The model under review builds one solid part; all positions refer to its coordinate system, in mm. Face numbers are marked on the shaded views. A direction names the side the tool comes from. Round coordinates to 2 decimals unless told otherwise and drop trailing zeros. Order: outer loops, then holes, each group sorted by start corner. A loop starts at its lowest first (then second) coordinate and runs counter-clockwise, first axis right, second up. Notation, with made-up numbers: (41, 53) -> (50, 53) arc R21 ccw to (50, 60) -> close; hole circle Ø4 at (23.25, -15.5). An arc over 180 degrees is marked (long way). Return JSON: item names as keys, results as strings. Group by question number.
Autodesk Inventor part; units mm, degrees
ref_plane "YZ Plane" through (0, 0, 0) normal (1, 0, 0) x (0, 1, 0)
ref_plane "XZ Plane" through (0, 0, 0) normal (0, 1, 0) x (-1, 0, 0)
ref_plane "XY Plane" through (0, 0, 0) normal (0, 0, 1) x (1, 0, 0)
sketch "Skizze1" plane through (0, 0, 0) normal (0, 1, 0) x (-1, 0, 0)
  line L0 (0, -50) -> (-50, -50)
  line L1 (-50, -50) -> (-50, 50)
  line L2 (-50, 50) -> (0, 50)
  line L3 (0, -50) -> (50, -50)
  line L4 (50, -50) -> (50, 50)
  line L5 (50, 50) -> (0, 50)
  line L6 (-122.5, 0) -> (122.5, 0) construction
  line L7 (0, -77.2) -> (0, 113.2) construction
  dimension "d1" = 100
  dimension "d3" = 100
extrude "Grundkoerper" add sketch "Skizze1" along normal mid plane 65
sketch "Skizze2" plane through (0, -32.5, 0) normal (0, -1, 0) x (1, 0, 0)
  line L0 (-50, -50) -> (50, -50)
  line L1 (50, 50) -> (-50, 50)
  point P0 (0, 0)
  point P1 (0, 0)
  point P2 (-87.5, 0)
  point P3 (87.5, 0)
  dimension "d8" = 0
sketch "Skizze3" plane through (0, 0, 0) normal (1, 0, 0) x (0, 1, 0)
  line L0 (49, 0) -> (-49, 0) construction
  line L1 (-32.5, 50) -> (-32.5, -50) construction
  line L2 (32.5, -50) -> (32.5, 50) construction
  line L3 (32.5, 36) -> (-12.5, 36)
  line L4 (-12.5, 36) -> (-12.5, 32.25)
  line L5 (-17.5, 18) -> (-32.5, 18)
  line L6 (-32.5, -50) -> (-32.5, 50)
  line L7 (-32.5, 18) -> (-32.5, 0)
  line L8 (-32.5, 0) -> (32.5, 0)
  line L9 (32.5, 0) -> (32.5, 36)
  line L10 (-12.5, 32.25) -> (-17.5, 32.25)
  line L11 (-17.5, 32.25) -> (-17.5, 18)
  point P0 (0, 0)
  dimension "d9" = 45
  dimension "d10" = 72
  dimension "d11" = 36
  dimension "d33" = 5
  dimension "d34" = 64.5
revolve "Lagersitz" cut sketch "Skizze3" angle 360 about axis through (0, -32.5, 0) along (0, -1, 0)
sketch "Skizze_Lagersitz" plane through (0, 0, 0) normal (1, 0, 0) x (0, 1, 0)
  line L0 (-12.5, 36) -> (32.5, 36)
  line L1 (-12.5, -36) -> (-12.5, 36)
  line L2 (-17.5, 32.25) -> (-12.5, 32.25)
  line L3 (-17.5, -32.25) -> (-17.5, 32.25)
  line L4 (-32.5, 18) -> (-17.5, 18)
  line L5 (-32.5, -18) -> (-17.5, -18)
  line L6 (-17.5, -32.25) -> (-12.5, -32.25)
  line L7 (-12.5, -36) -> (32.5, -36)
  line L8 (32.5, 36) -> (32.5, -36)
  line L9 (32.5, 50) -> (32.5, -50)
  line L10 (30, -50) -> (30, 0)
  line L11 (-32.5, -18) -> (-32.5, 18)
  line L12 (-32.5, 50) -> (-32.5, -50)
  line L13 (-32.5, -50) -> (-32.5, 50)
  line L14 (-12.5, -36) -> (-12.5, 36)
  point P0 (0, 0)
  point P1 (30, 86)
  point P2 (30, 14)
  point P3 (-30, 32)
  point P4 (-30, 68)
sketch "Skizze10" plane through (0, 0, 0) normal (1, 0, 0) x (0, 1, 0)
  line L0 (49, 0) -> (-49, 0)
  line L1 (-32.5, 18) -> (-17.5, 18) construction
  line L2 (-32.5, -50) -> (-32.5, 50) construction
  line L3 (-17.5, -32.25) -> (-17.5, 32.25) construction
  line L4 (-32.5, 50) -> (-32.5, -50)
  line L5 (-29.5, 27.5) -> (-21.7, 27.5)
  line L6 (-21.2, 27) -> (-21.2, 22.5)
  line L7 (-21.2, 22.5) -> (-17.5, 22.5)
  line L8 (-17.5, 22.5) -> (-17.5, 18)
  line L9 (-32.5, 40) -> (-32.5, 0)
  line L10 (-32.5, 0) -> (-17.5, 0)
  line L11 (-17.5, 0) -> (-17.5, 22.5)
  arc A0 (-21.2, 27) -> (-21.7, 27.5) centre (-21.7, 27) ccw
  line L12 (-29.5, 27.5) -> (-29.5, 40)
  line L13 (-29.5, 40) -> (-32.5, 40)
  point P0 (0, 0)
  dimension "d117" = 55
  dimension "d118" = 0.5
  dimension "d119" = 45
  dimension "d124" = 8.3
  dimension "d125" = 3
  dimension "d126" = 80
revolve "RWDR" cut sketch "Skizze10" angle 360 about axis through (0, -32.5, 0) along (0, -1, 0)
sketch "Skizze_RWDR" plane through (0, 0, 0) normal (1, 0, 0) x (0, 1, 0)
  line L0 (-32.5, -40) -> (-32.5, 40)
  line L1 (-32.5, 40) -> (-29.5, 40)
  line L2 (-29.5, -40) -> (-29.5, 40)
  line L3 (-32.5, -40) -> (-29.5, -40)
  line L4 (-29.5, 27.5) -> (-21.7, 27.5)
  line L5 (-21.2, -27) -> (-21.2, 27)
  line L6 (-29.5, -27.5) -> (-21.7, -27.5)
  arc A0 (-21.7, -27.5) -> (-21.2, -27) centre (-21.7, -27) ccw
  arc A1 (-21.2, 27) -> (-21.7, 27.5) centre (-21.7, 27) ccw
  line L7 (-21.2, 22.5) -> (-17.5, 22.5)
  line L8 (-21.2, -22.5) -> (-17.5, -22.5)
  line L9 (-17.5, 22.5) -> (-17.5, -22.5)
  point P0 (0, 0)
sketch "Skizze5" plane through (0, 32.5, 0) normal (0, 1, 0) x (1, 0, 0)
  circle A0 centre (0, 0) radius 36 construction
  circle A1 centre (0, 0) radius 43 construction
  line L0 (-50, -50) -> (50, -50) construction
  line L1 (50, 50) -> (-50, 50)
  line L2 (-50, 50) -> (50, 50) construction
  line L3 (0, 77.2) -> (0, -113.2) construction
  line L4 (0, 0) -> (21.5, -37.2391) construction
  point P0 (43, 0)
  point P1 (21.5, 37.2391)
  point P2 (-21.5, 37.2391)
  point P3 (-43, 0)
  point P4 (-21.5, -37.2391)
  dimension "d40" = 86
  dimension "d38" = 100
  dimension "d39" = 72
  dimension "d110" = 30
  dimension "d114" = 360
hole "M6_Boh_Lagerpresse" at (21.5, 32.5, 37.2391) at (43, 32.5, 0) at (21.5, 32.5, -37.2391) at (-21.5, 32.5, -37.2391) at (-43, 32.5, 0) at (-21.5, 32.5, 37.2391) direction (0, -1, 0) diameter 4.917 depth 17.1 tip angle 118 countersink diameter 6 countersink angle 90
sketch "Skizze11" plane through (0, -29.5, 0) normal (0, -1, 0) x (1, 0, 0)
  circle A0 centre (0, 0) radius 40 construction
  circle A1 centre (0, 0) radius 27.5 construction
  circle A2 centre (0, 0) radius 33.75 construction
  line L0 (0, 113.2) -> (0, -77.2) construction
  line L1 (-122.5, 0) -> (122.5, 0)
  point P0 (0, 33.75)
  point P1 (-33.75, 0)
  point P2 (0, -33.75)
  point P3 (33.75, 0)
  dimension "d129" = 67.5
  dimension "d127" = 55
  dimension "d128" = 80
  dimension "d132" = 360
hole "M3_RWDR_Fixierung" at (0, -29.5, 33.75) at (-33.75, -29.5, 0) at (0, -29.5, -33.75) at (33.75, -29.5, 0) direction (0, 1, 0) diameter 2.459 depth 8.8 tip angle 118 countersink diameter 3 countersink angle 90
sketch "Skizze8" plane through (50, 32.5, -50) normal (0, 0, -1) x (-1, 0, 0)
  line L0 (0, 0) -> (100, 0) construction
  line L1 (100, -65) -> (0, -65) construction
  line L2 (0, 0) -> (0, -65) construction
  line L3 (100, 0) -> (100, -65) construction
  line L4 (50, -84.5) -> (50, 17) construction
  line L5 (-72.5, -32.5) -> (172.5, -32.5) construction
  point P0 (50, -32.5)
  point P1 (25, -16.25)
  point P2 (75, -16.25)
  point P3 (25, -48.75)
  point P4 (75, -48.75)
  dimension "d81" = 100
  dimension "d82" = 50
  dimension "d83" = 65
  dimension "d84" = 32.5
hole "M8_Boh_Fixierung_1" at (25, 16.25, -50) at (-25, 16.25, -50) at (25, -16.25, -50) at (-25, -16.25, -50) direction (0, 0, 1) diameter 6.647 depth 18.2 tip angle 118 countersink diameter 8 countersink angle 90
sketch "Skizze9" plane through (50, -32.5, -50) normal (1, 0, 0) x (0, 0, -1)
  line L0 (-50, 81.5) -> (-50, -16.5) construction
  line L1 (0, 65) -> (0, 0) construction
  line L2 (-100, 65) -> (0, 65) construction
  line L3 (0, 0) -> (-100, 0) construction
  line L4 (-163.2, 32.5) -> (27.2, 32.5) construction
  point P0 (-50, 32.5)
  point P1 (-25, 16.25)
  point P2 (-25, 48.75)
  dimension "d92" = 32.5
  dimension "d93" = 65
  dimension "d94" = 50
  dimension "d95" = 25
hole "M8_Boh_Fixierung_2" at (50, -16.25, -25) at (50, 16.25, -25) direction (-1, 0, 0) diameter 6.647 depth 18.2 tip angle 118 countersink diameter 8 countersink angle 90
mirror "M8_Boh_Fixierung_2_Spiegel" about plane through (0, 0, 0) normal (1, 0, 0) of "M8_Boh_Fixierung_2"
chamfer "Fase_Lagersitz" distance 0.25 angle 45 1 edges at (0, -12.5, -32.25)
chamfer "Fase_Deckel" distance 1 angle 45 1 edges at (0, 32.5, -36)
chamfer "Fase_Allgemein" distance 2.5 angle 45 4 edges at (50, 0, 50) (-50, 0, 50) (50, 0, -50) (-50, 0, -50)
chamfer "Fase_RWDR" distance 0.2 angle 45 2 edges at (0, -29.5, -27.5) (0, -32.5, -40)
equation "\"d40\" = 0.5 * d38 + 0.5 * d39"
equation "\"d129\" = 0.5 * d128 + 0.5 * d127"
properties part number "200-10-ROCKER-BEARING-01" material "Aluminium 6061"
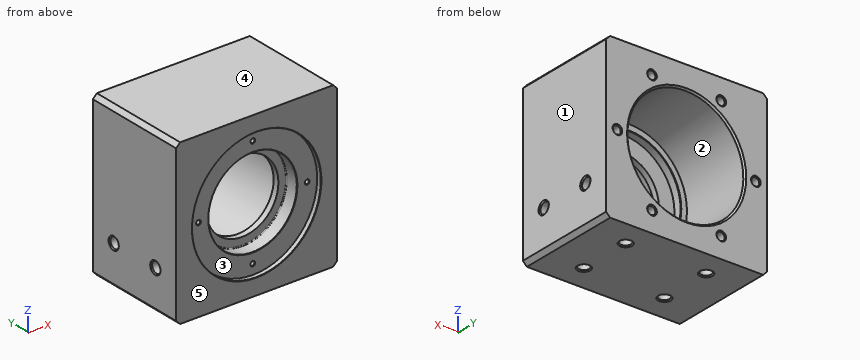
Item 1: The part is to be moulded in two halves that separate along Z. For the marked faces 3, 4 and 5, say which applies: +Z half, -Z half, draft (parallel to the pull), parting line (faces both ways), or undercut.
Item 2: For the marked faces 1 and 2, list the 3-axis set-ups (+Z, -Z, +X, -X, +Y, -Y) from which the entire face can be reached by the end or side of a thin tool; tool diameter is ignored.
Item 3: Insertion check: pin 1 Ø6 at (x, y) = (-25, 16.25) entering from -Z; pin 2 Ø4.5 at (x, z) = (21.5, 37.24) entering from +Y; pin 3 Ø10 at (x, z) = (26.5, -29) entering from -Y; pin 4 Ø4 at (y, z) = (-16.25, -25) entering from +X. Each pin has a flat end and moves straight along its axis. Give the tip position at first contact, or say it passes through.
Item 4: Consider section A-A on y = 28.5. State the section outline as (x, z) points.
Item 5: Wall thickness on line 1 along Y through (x, z) = (-25, -42); line 2 along X through (y, z) = (16, -40); line 3 along Z through (x, y) = (0, -29): over which ranges is each line inside the solid? List them lowest first.
Item 6: Consider section B-B on y = 4. State the section outline as (x, z) points, plus the area to 3 significant figures.
Values:
{
 "1": {"face 3": "undercut", "face 4": "+Z half", "face 5": "draft"},
 "2": {"face 1": "+Z, -Z, +X, +Y, -Y", "face 2": "+Y"},
 "3": {"pin 1": "z = -31.61", "pin 2": "y = 15.28", "pin 3": "y = -32.5", "pin 4": "x = 31"},
 "4": {"outline": "(-50, -47.5) -> (-47.5, -50) -> (47.5, -50) -> (50, -47.5) -> (50, 47.5) -> (47.5, 50) -> (-47.5, 50) -> (-50, 47.5) -> close; hole circle Ø4.92 at (-43, 0); hole circle Ø72 at (0, 0); hole circle Ø4.92 at (-21.5, -37.24); hole circle Ø4.92 at (-21.5, 37.24); hole circle Ø4.92 at (21.5, -37.24); hole circle Ø4.92 at (21.5, 37.24); hole circle Ø4.92 at (43, 0)"},
 "5": {"line 1": "-32.5 to -19.57, -12.93 to 12.93, 19.57 to 32.5", "line 2": "-50 to -28.31, -21.69 to 21.69, 28.31 to 50", "line 3": "-50 to -34.98, -32.52 to -27.5, 27.5 to 32.52, 34.98 to 50"},
 "6": {"outline": "(-50, -47.5) -> (-47.5, -50) -> (47.5, -50) -> (50, -47.5) -> (50, 47.5) -> (47.5, 50) -> (-47.5, 50) -> (-50, 47.5) -> close; hole circle Ø72 at (0, 0)", "area": "5,920 mm^2"}
}
